```python
from build123d import *

# Parameters (mm, degrees)
SKETCH1_W           = 6
SKETCH1_H           = 5
BOSS_EXTRUDE1_DEPTH = 2
BOSS_EXTRUDE2_DEPTH = 2
CUT_EXTRUDE1_DEPTH  = 10


with BuildPart() as part:
    # Sketch1 → Boss-Extrude1 (new body)
    with BuildSketch(Plane.XY):
        with Locations((3, 2.5)):
            Rectangle(SKETCH1_W, SKETCH1_H)
    extrude(amount=BOSS_EXTRUDE1_DEPTH)

    # Sketch2 → Boss-Extrude2 (add)
    with BuildSketch(Plane.XY.offset(2)):
        Polygon((0, 0), (0, 2), (4, 2), (6, 0), align=None)
    extrude(amount=BOSS_EXTRUDE2_DEPTH)

    # 3DSketch1 → Cut-Extrude1 (cut, along a direction that is not the sketch's normal)
    with BuildSketch(Plane(origin=(5, 0, 2), x_dir=(-0.727606875108999, 0.485071250072666, 0.485071250072666), z_dir=(0.6666666666666666, 0.3333333333333333, 0.6666666666666666))):
        Polygon((0, 0), (2.42535625, 1.45521375), (4.123105626, 0), (1.697749375, -1.45521375), align=None)
    extrude(amount=CUT_EXTRUDE1_DEPTH, dir=(1, 0, 0), mode=Mode.SUBTRACT)


solid = part.part
```
Check sheet for the modelled part. Datum: model origin and axes. Units: mm. A direction names the side the tool comes from. Give positions to 0.01 mm unless a question says otherwise; leave off trailing zeros. Loops run counter-clockwise (first coordinate to the right, second up) from the corner with the lowest first, then second, coordinate; pieces in that order, holes last. Notation, with made-up numbers: M 23,19 L 76,19 A17 cw 76,24 Z; hole C -9,7 d8. An arc over 180 degrees is marked long. Answer as CSV lines item,"result".
Item 1: Scan lines: L1, parallel to Z at x = 3, y = 3.6; L2, parallel to Y at x = 3.45, z = 3. Record each from-to range of solid material in increasing order.
Reply:
L1,"0 to 2"
L2,"0 to 1.1"
Item 2: Sectioned sample at D-D, the plane x = 4.8. Enter the section's corners in (y, z), then the cut area to 3 significant figures.
Reply:
outline,"M 0,0 L 5,0 L 5,2 L 0.4,2 L 0,2.2 Z"
area,"10.0 mm^2"
Item 3: Set-up check for faces 1 (the face through (4, 3, 2)), 2 (the face through (2, 2, 3)), 3 (the face through (0, 1.9, 1.5)): record each of +Z, -Z, +X, -X, +Y, -Y from which the full face is reachable in a straight line by a thin tool's end or side.
Reply:
face 1,"+Z, +X, +Y"
face 2,"+Z, +X, -X, +Y"
face 3,"+Z, -Z, -X, +Y, -Y"
Item 4: Sectioned sample at C-C, the plane z = 2.3. Enter the section's corners in (x, y).
Reply:
outline,"M 0,0 L 4.7,0 L 3.7,2 L 0,2 Z"
Item 5: Sectioned sample at B-B, the plane y = 1.5. Enter the section's corners in (x, z), then the cut area to 3 significant figures.
Reply:
outline,"M 0,0 L 6,0 L 6,2 L 4.25,2 L 2.25,4 L 0,4 Z"
area,"18.5 mm^2"
Item 6: Depth check by flat-ended pin: pin 1 Ø0.6 at (x, z) = (2.5, 3) entering from +Y; pin 2 Ø1.5 at (x, z) = (5.5, 3) entering from -Y; pin 3 Ø1 at (y, z) = (1.5, 3) entering from +X. Enter the tip coordinate at first touch or a pass-through.
Reply:
pin 1,"y = 2"
pin 2,"through"
pin 3,"x = 3.81"
Item 7: Sectioned sample at A-A, the plane x = 1.25. Enter the section's corners in (y, z), then the cut area to 3 significant figures.
Reply:
outline,"M 0,0 L 5,0 L 5,2 L 2,2 L 2,4 L 0,4 Z"
area,"14.0 mm^2"
